Answer from the drawing. Dimensions are ordinates in mm from the lowest x, y and z of the part. A direction names the side the tool comes from. Coordinates: 2 decimals unless noted, no trailing zeros. Order: outer loops, then holes, each group sorted by start corner. A loop starts at its lowest first (then second) coordinate and runs counter-clockwise, first axis right, second up. Notation, with made-up numbers: (31, 26) - (35, 26) arc R8 ccw to (35, 36) - close; hole circle Ø10 at (24, 28). An arc over 180 degrees is marked (long way). Use a Markdown table: item, result. Add a question column.
Item 1: The part is cut by section A-A, the plane x = 39. Give the vertices of the cut face in (y, z) (3 decimals).
Item 2: Flat-ended cylindrical pins translate along their axes: P1, Ø12, axis at y = 20.5, z = 23, coming from the -X side; P2, Ø1.5, axis at x = 13, z = 29.5, coming from the +Y side. Find the tip coordinate at first contact, or state that the pin passes through.
Item 3: The part is cut by section B-B, the plane z = 25.5. Give the vertices of the cut face in (x, y) (3 decimals).
Item 4: The part is cut by section C-C, the plane y = 3.5. State how many separate pieces and enclosed holes the cut face has, then the cut area to 3 significant figures.
Item 5: For the marked faces 1 and 2, determine the directions among +Z, -Z, +X, -X, +Y, -Y from which every point of the face is accessible in a straight line to the end or side of a thin tool.
Item 6: The part is cut by section D-D, the plane z = 33. Give the vertices of the cut face in (x, y), then the cut area to 3 significant figures.
Item 7: Find the intervals of material crossed by line 1 along Z through (x, y) = (39, 7.75) (3 decimals); line 2 along Z through (x, y) = (36.5, 2) (1 decimal); line 3 along Y through (x, z) = (24.5, 41), in increasing order.
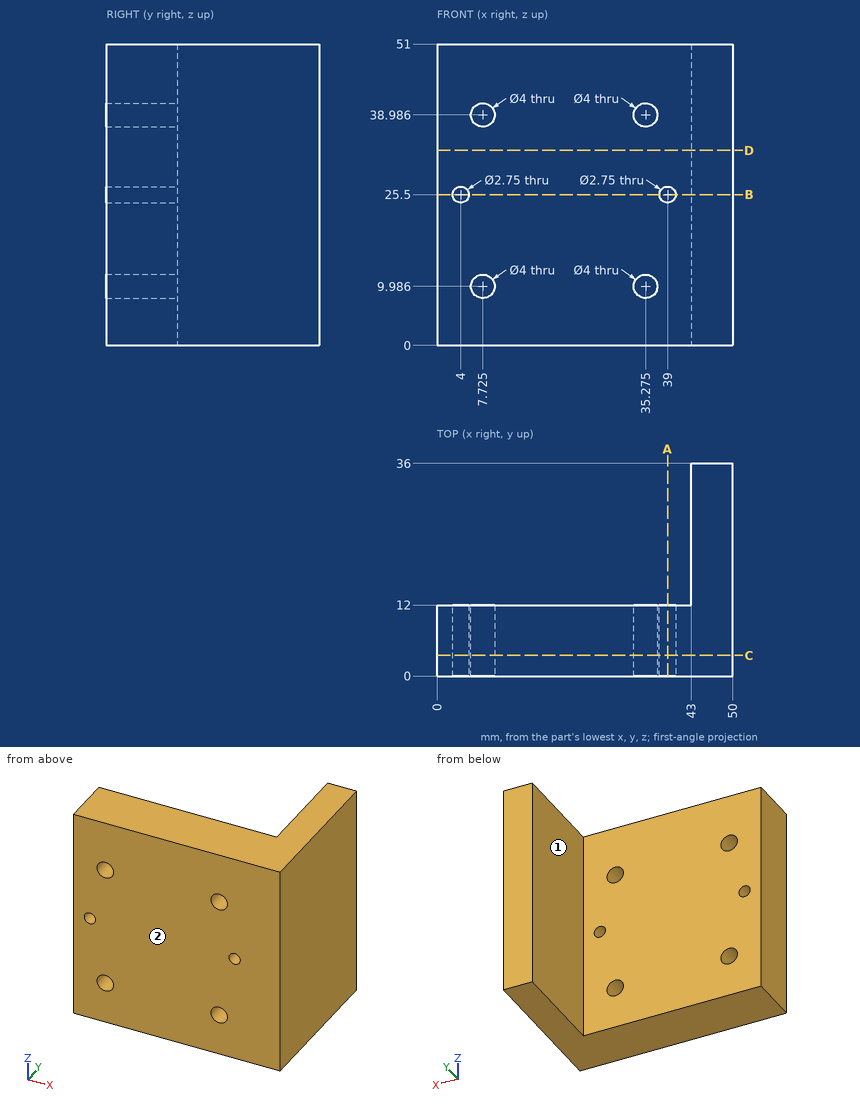
Solution:
| question | item | result |
|---|---|---|
| 1 | outline | (0, 0) - (12, 0) - (12, 24.125) - (0, 24.125) - close; (0, 26.875) - (12, 26.875) - (12, 51) - (0, 51) - close |
| 2 | P1 | stops at x = 43 |
| 2 | P2 | stops at y = 12 |
| 3 | outline | (0, 0) - (2.625, 0) - (2.625, 12) - (0, 12) - close; (5.375, 0) - (37.625, 0) - (37.625, 12) - (5.375, 12) - close; (40.375, 0) - (50, 0) - (50, 36) - (43, 36) - (43, 12) - (40.375, 12) - close |
| 4 | separate pieces | 1 |
| 4 | enclosed holes | 6 |
| 4 | area | 2,490 mm2 |
| 5 | face 1 | +Z, -Z, -X, +Y |
| 5 | face 2 | +Z, -Z, +X, -X, -Y |
| 6 | outline | (0, 0) - (50, 0) - (50, 36) - (43, 36) - (43, 12) - (0, 12) - close |
| 6 | area | 768 mm2 |
| 7 | line 1 | z = 0 to 24.125, 26.875 to 51 |
| 7 | line 2 | z = 0 to 8.4, 11.6 to 37.4, 40.6 to 51 |
| 7 | line 3 | y = 0 to 12 |
